Design review of the part built by this model. Coordinates are the model's own, in mm. Face numbers are marked on the shaded views. A direction names the side the tool comes from. Coordinates: 2 decimals unless noted, no trailing zeros. Order: outer loops, then holes, each group sorted by start corner. A loop starts at its lowest first (then second) coordinate and runs counter-clockwise, first axis right, second up. Notation, with made-up numbers: (10.25, 33) -> (29.25, 33) arc R30 cw to (29.25, 62) -> close; hole circle Ø5 at (-11.75, 24). An arc over 180 degrees is marked (long way). Write item = value, one per line.
Autodesk Inventor part; units mm, degrees
ref_plane "YZ Plane" through (0, 0, 0) normal (1, 0, 0) x (0, 1, 0)
ref_plane "XZ Plane" through (0, 0, 0) normal (0, 1, 0) x (-1, 0, 0)
ref_plane "XY Plane" through (0, 0, 0) normal (0, 0, 1) x (1, 0, 0)
sketch "Эскиз1" plane through (0, 0, 0) normal (0, 1, 0) x (-1, 0, 0)
  line L0 (12.75, -5) -> (-12.75, -5)
  line L1 (-12.75, -5) -> (-12.75, 5)
  line L2 (-12.75, 5) -> (12.75, 5)
  line L3 (12.75, 5) -> (12.75, -5)
  line L4 (-12.75, -5) -> (12.75, 5) construction
  line L5 (12.75, -5) -> (-12.75, 5) construction
  line L6 (-10.75, -3) -> (10.75, -3)
  line L7 (10.75, -3) -> (10.75, 3)
  line L8 (10.75, 3) -> (-10.75, 3)
  line L9 (-10.75, 3) -> (-10.75, -3)
  point P0 (0, 0)
  point P1 (0, 0)
  dimension "d0" = 25.5
  dimension "d1" = 10
  dimension "d2" = 2
extrude "Выдавливание1" add sketch "Эскиз1" along normal blind 82.9
sketch "Эскиз3" plane through (12.75, 0, -5) normal (0, 0, -1) x (-1, 0, 0)
  line L0 (0, 0) -> (0, 82.9)
  line L1 (25.5, 0) -> (25.5, 82.9)
  line L2 (25.5, 0) -> (25.5, 82.9)
  line L3 (0, 0) -> (0, 82.9)
  line L4 (0, 82.9) -> (25.5, 82.9)
  arc A0 (2, 72.9) -> (23.5, 72.9) centre (12.75, 72.9) ccw
  line L5 (23.5, 0) -> (23.5, 82.9)
  line L6 (2, 0) -> (2, 82.9)
  line L7 (23.5, 0) -> (23.5, 82.9)
  line L8 (23.5, 72.9) -> (23.5, 82.9)
  line L9 (23.5, 82.9) -> (2, 82.9)
  line L10 (2, 72.9) -> (2, 82.9)
  point P0 (12.75, 0)
  dimension "d10" = 10
extrude "Выдавливание3" cut sketch "Эскиз3" against normal up to surface (2 mm away)
sketch "Эскиз2" plane through (12.75, 0, 5) normal (1, 0, 0) x (0, 0, -1)
  line L0 (0, 82.9) -> (10, 82.9) construction
  line L1 (10, 82.9) -> (0, 72.9) construction
  line L2 (0, 0) -> (0, 82.9) construction
  line L3 (0, 82.9) -> (10, 72.9) construction
  line L4 (10, 0) -> (10, 82.9) construction
  line L5 (10, 0) -> (0, 10) construction
  line L6 (0, 0) -> (10, 10) construction
  circle A0 centre (5, 77.9) radius 0.5
  circle A1 centre (5, 5) radius 0.5
  point P0 (5, 0)
  dimension "d5" = 1
  dimension "d6" = 1
hole "Отверстие1" at (12.75, 77.9, 0) at (12.75, 5, 0) direction (-1, 0, 0) diameter 1 depth 2 countersink diameter 1.5 countersink angle 90
mirror "Зеркальное отражение1" about plane through (0, 0, 0) normal (1, 0, 0) of "Отверстие1"
properties part number "board-1-new"
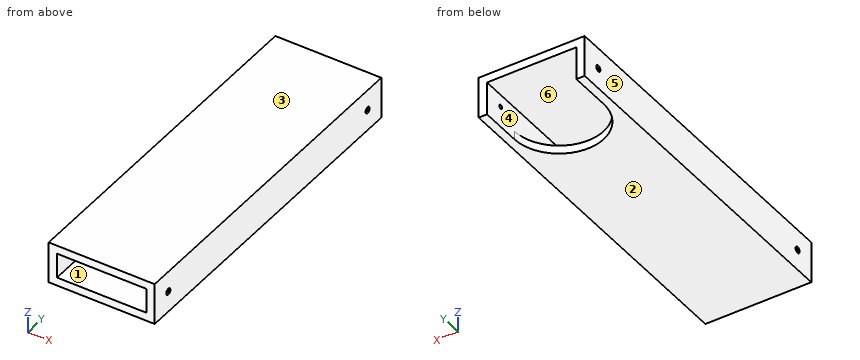
(1) The part is to be moulded in two halves that separate along Z. For the marked faces 1, 2, 3 and 4, say which applies: released by +Z, released by -Z, zero draft, split by the parting line, or undercut.
Report:
face_1 = undercut
face_2 = released by -Z
face_3 = released by +Z
face_4 = undercut
(2) For L1, parallel to Y at x = -11.25, z = 0; L2, parallel to Z at x = -11.05, y = 5; L3, parallel to X at y = 6, z = -2, list the stretches that pass through material, from the lowest coordinate up.
Report:
L1 = 0 to 4.5, 5.5 to 77.4, 78.4 to 82.9
L2 = -5 to -0.5, 0.5 to 5
L3 = -12.75 to -10.75, 10.75 to 12.75
(3) We need section A-A (x = 0). Write out the cut boundary in (y, z).
Report:
outline = (0, -5) -> (62.15, -5) -> (62.15, -3) -> (0, -3) -> close; (0, 3) -> (82.9, 3) -> (82.9, 5) -> (0, 5) -> close
(4) We need section D-D (y = 70). Write out the cut boundary in (x, z).
Report:
outline = (-12.75, -5) -> (-10.35, -5) -> (-10.35, -3) -> (-10.75, -3) -> (-10.75, 3) -> (10.75, 3) -> (10.75, -3) -> (10.35, -3) -> (10.35, -5) -> (12.75, -5) -> (12.75, 5) -> (-12.75, 5) -> close
(5) For the marked faces 5 and 6, list the 3-axis set-ups (+Z, -Z, +X, -X, +Y, -Y) from which the entire face can be reached by the end or side of a thin tool; tool diameter is ignored.
Report:
face_5 = +Z, -Z, -X, +Y, -Y
face_6 = +Y, -Y
(6) We need section C-C (z = -4). Write out the cut boundary in (x, y), and give its area (3 significant figures).
Report:
outline = (-12.75, 0) -> (12.75, 0) -> (12.75, 82.9) -> (10.75, 82.9) -> (10.75, 72.9) arc R10.75 cw to (-10.75, 72.9) -> (-10.75, 82.9) -> (-12.75, 82.9) -> close
area = 1,720 mm²
(7) Insertion check: pin 1 (6 mm diameter, centred on x = -3, z = -2.5, fed in from +Y). The pin has a flat end and moves straight along its axis. Give the tip position at first contact, or say it passes through.
Report:
pin_1 = 63.95
(8) We need section B-B (y = 50). Write out the cut boundary in (x, z).
Report:
outline = (-12.75, -5) -> (12.75, -5) -> (12.75, 5) -> (-12.75, 5) -> close; hole (-10.75, -3) -> (10.75, -3) -> (10.75, 3) -> (-10.75, 3) -> close
